Build history of the part. All positions in model axes, mm. Face numbers are marked on the shaded views. A direction names the side the tool comes from. Give positions to 0.01 mm unless a question says otherwise; leave off trailing zeros. Loops run counter-clockwise (first coordinate to the right, second up) from the corner with the lowest first, then second, coordinate; pieces in that order, holes last. Notation, with made-up numbers: (33, 38.25) - (42, 38.25) arc R13 ccw to (42, 62.25) - close; hole circle Ø10 at (36, 17.25). An arc over 180 degrees is marked (long way). Return JSON: item names as keys, results as strings. Group by question number.
1) Slice it at B-B (x = 0). List the corners of the cut face in (y, z).
2) Slice it at A-A (z = 0). List the corners of the cut face in (x, y).
3) Mould opens along Z. For the marked faces 1, 2 and 3 say: released by +Z, released by -Z, zero draft, split by the parting line, or undercut.
4) Drop flat-ended pins along their axis: pin 1 (3 mm diameter, centred on x = 3.5, z = 2.5, fed in from +Y); pin 2 (1.2 mm diameter, centred on x = -0.5, z = -0.5, fed in from -Y). Give the stop position or say it passes through.
5) Slice it at C-C (y = 2.1). List the corners of the cut face in (x, z), and give its area (3 significant figures).
6) 3-axis set-ups, long thin cutter, end or side, ignore diameter. For the marked faces 4 and 5: which of +Z, -Z, +X, -X, +Y, -Y reach the whole face in a straight line?
7) Drill centre lines: probe 1 along X at (y, z) = (1.6, 0); probe 2 along Z at (x, y) = (0.5, 2.25); probe 3 along Z at (x, y) = (0.75, 1.15). Where is each one in solid material? Low to high. Write a range as from..to.
8) Slice it at D-D (y = 3.45). List the corners of the cut face in (x, z).
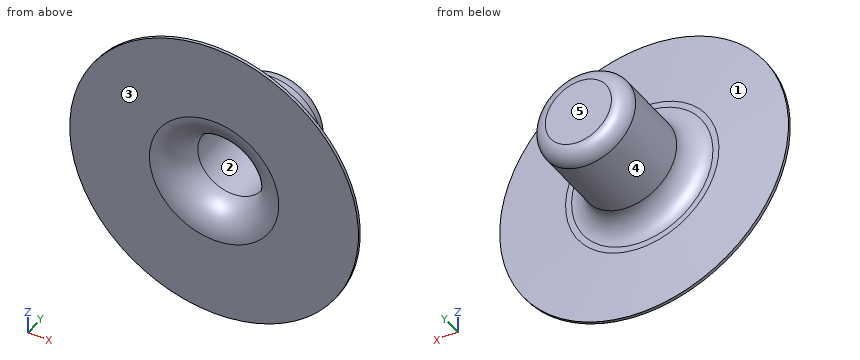
```python
from build123d import *

# Parameters (mm, degrees)
CROQUIS1_R              = 4.8
SALIENTE_EXTRUIR1_DEPTH = 0.2
CROQUIS2_R              = 1.6
SALIENTE_EXTRUIR2_DEPTH = 3.5
REDONDEO1_R             = 0.5
REDONDEO2_R             = 0.75
CROQUIS3_R              = 1.15
CORTAR_EXTRUIR1_DEPTH   = 3
REDONDEO3_R             = 1
CHAFL_N1_SIZE           = 0.1
CHAFL_N1_SIZE2          = 2.25


with BuildPart() as part:
    # Croquis1 → Saliente-Extruir1 (new body)
    with BuildSketch(Plane(origin=(0, 0, 0), x_dir=(1, 0, 0), z_dir=(0, 1, 0))):
        with Locations(Location((0, 0, 0), (0, 0, 270))):
            Circle(CROQUIS1_R)
    extrude(amount=SALIENTE_EXTRUIR1_DEPTH)

    # Croquis2 → Saliente-Extruir2 (add)
    with BuildSketch(Plane(origin=(0, 0.2, 0), x_dir=(1, 0, 0), z_dir=(0, 1, 0))):
        with Locations(Location((0, 0, 0), (0, 0, 270))):
            Circle(CROQUIS2_R)
    extrude(amount=SALIENTE_EXTRUIR2_DEPTH)

    # Redondeo1
    redondeo1_edges = [part.edges().sort_by_distance(p)[0] for p in [
        (0, 3.7, -1.6),
    ]]
    fillet(redondeo1_edges, radius=REDONDEO1_R)

    # Redondeo2
    redondeo2_edges = [part.edges().sort_by_distance(p)[0] for p in [
        (0, 0.2, -1.6),
    ]]
    fillet(redondeo2_edges, radius=REDONDEO2_R)

    # Croquis3 → Cortar-Extruir1 (cut)
    with BuildSketch(Plane.XZ):
        with Locations(Location((0, 0, 0), (0, 0, 270))):
            Circle(CROQUIS3_R)
    extrude(amount=-CORTAR_EXTRUIR1_DEPTH, mode=Mode.SUBTRACT)

    # Redondeo3
    redondeo3_edges = [part.edges().sort_by_distance(p)[0] for p in [
        (0, 0, 1.15),
    ]]
    fillet(redondeo3_edges, radius=REDONDEO3_R)

    # Chaflán1
    chafl_n1_edges = [part.edges().sort_by_distance(p)[0] for p in [
        (0, 0.2, -4.8),
    ]]
    chafl_n1_side = [part.faces().sort_by_distance(p)[0] for p in [
        (0, 0.1, -4.8),
    ]]
    chamfer(chafl_n1_edges, length=CHAFL_N1_SIZE, length2=CHAFL_N1_SIZE2, reference=chafl_n1_side[0])


solid = part.part
```
Results:
{
 "1": {"outline": "(0, -4.8) - (0.1, -4.8) - (0.2, -2.55) - (0.2, -2.35) arc R0.75 cw to (0.95, -1.6) - (3.2, -1.6) arc R0.5 ccw to (3.7, -1.1) - (3.7, 1.1) arc R0.5 ccw to (3.2, 1.6) - (0.95, 1.6) arc R0.75 cw to (0.2, 2.35) - (0.2, 2.55) - (0.1, 4.8) - (0, 4.8) - (0, 2.15) arc R1 ccw to (1, 1.15) - (3, 1.15) - (3, -1.15) - (1, -1.15) arc R1 ccw to (0, -2.15) - close"},
 "2": {"outline": "(-4.8, 0) - (-2.15, 0) arc R1 ccw to (-1.15, 1) - (-1.15, 3) - (1.15, 3) - (1.15, 1) arc R1 ccw to (2.15, 0) - (4.8, 0) - (4.8, 0.1) - (2.55, 0.2) - (2.35, 0.2) arc R0.75 cw to (1.6, 0.95) - (1.6, 3.2) arc R0.5 ccw to (1.1, 3.7) - (-1.1, 3.7) arc R0.5 ccw to (-1.6, 3.2) - (-1.6, 0.95) arc R0.75 cw to (-2.35, 0.2) - (-2.55, 0.2) - (-4.8, 0.1) - close"},
 "3": {"face 1": "split by the parting line", "face 2": "undercut", "face 3": "zero draft"},
 "4": {"pin 1": "y = 0.19", "pin 2": "y = 0.46"},
 "5": {"outline": "circle Ø3.2 at (0, 0); hole circle Ø2.3 at (0, 0)", "area": "3.89 mm2"},
 "6": {"face 4": "+Y", "face 5": "+Z, -Z, +X, -X, +Y"},
 "7": {"probe 1": "-1.6..-1.15, 1.15..1.6", "probe 2": "-1.52..-1.04, 1.04..1.52", "probe 3": "-1.41..-0.87, 0.87..1.41"},
 "8": {"outline": "circle Ø3.07 at (0, 0)"}
}
